```python
from build123d import *

# Parameters (mm, degrees)
SKETCH1_R           = 1.75
BOSS_EXTRUDE1_DEPTH = 5
FILLET1_R           = 5
CUT_EXTRUDE1_DEPTH  = 10
SKETCH3_R           = 1.75
CUT_EXTRUDE2_DEPTH  = 10


with BuildPart() as part:
    # Sketch1 → Boss-Extrude1 (new body)
    with BuildSketch(Plane(origin=(0, 0, 0), x_dir=(1, 0, 0), z_dir=(0, 1, 0))):
        with BuildLine():
            Line((-15, 0), (-15, 50))
            ThreePointArc((-15, 50), (0, 65), (15, 50))
            Line((15, 50), (15, 0))
            ThreePointArc((15, 0), (0, -15), (-15, 0))
        make_face()
        Circle(SKETCH1_R, mode=Mode.SUBTRACT)
        with BuildLine():
            Line((12.25773045, 35.509501863), (8.623388818, 27.715631082))
            Line((8.623388818, 27.715631082), (10.414213562, 25.924806337))
            ThreePointArc((10.414213562, 25.924806337), (10.414213562, 23.096379213), (7.585786438, 23.096379213))
            Line((7.585786438, 23.096379213), (4.804718696, 25.877446954))
            ThreePointArc((4.804718696, 25.877446954), (4.249316753, 26.944364161), (4.406316685, 28.13689704))
            Line((4.406316685, 28.13689704), (8.632499302, 37.19997491))
            ThreePointArc((8.632499302, 37.19997491), (11.2903514, 38.167353961), (12.25773045, 35.509501863))
        make_face(mode=Mode.SUBTRACT)
    extrude(amount=BOSS_EXTRUDE1_DEPTH)

    # Fillet1
    fillet1_edges = [part.edges().sort_by_distance(p)[0] for p in [
        (8.623388818, 2.5, -27.715631082),
    ]]
    fillet(fillet1_edges, radius=FILLET1_R)

    # Sketch2 → Cut-Extrude1 (cut)
    with BuildSketch(Plane(origin=(0, 5, 0), x_dir=(1, 0, 0), z_dir=(0, 1, 0))):
        with BuildLine():
            Line((-15, 26.324644949), (-40.925594741, 69.238213195))
            Line((-40.925594741, 69.238213195), (-58.771967888, 111.080687023))
            Line((-58.771967888, 111.080687023), (39.28439299, 102.825794629))
            Line((39.28439299, 102.825794629), (15, 36.046990739))
            ThreePointArc((15, 36.046990739), (14.81014445, 39.245839168), (14.243243524, 42.399773179))
            ThreePointArc((14.243243524, 42.399773179), (11.621838426, 46.208407589), (7.127072402, 47.292169164))
            ThreePointArc((7.127072402, 47.292169164), (-0.175202385, 45.163669538), (-6.484026655, 40.9148504))
            ThreePointArc((-6.484026655, 40.9148504), (-11.826766868, 34.252893813), (-15, 26.324644949))
        make_face()
    extrude(amount=-CUT_EXTRUDE1_DEPTH, mode=Mode.SUBTRACT)

    # Sketch3 → Cut-Extrude2 (cut)
    with BuildSketch(Plane(origin=(0, 5, 0), x_dir=(1, 0, 0), z_dir=(0, 1, 0))):
        with Locations((-1.301778952, 33.126107378)):
            Circle(SKETCH3_R)
        with Locations((-2.207127715, 39.057409395)):
            Circle(SKETCH3_R)
        with Locations((-7.905919506, 31.519764857)):
            Circle(SKETCH3_R)
    extrude(amount=-CUT_EXTRUDE2_DEPTH, mode=Mode.SUBTRACT)


solid = part.part
```
The listing builds one solid part. Answer for the finished solid, in the listing's coordinates (mm). A direction names the side the tool comes from. Coordinates: 2 decimals unless noted, no trailing zeros. Write each loop counter-clockwise with the first axis right and the second up, starting at its lowest first coordinate (ties: lowest second). Pieces come first, ordered by that corner, then holes.
Q1. The mould has two halves that part along X. Classify faces 1 (the cylindrical face through (-1.53, 2.54, -34.86)), 2 (the flat face through (0, 0, -17)), 3 (the flat face through (-15, 2, -13)): released by +X, released by -X, zero draft, split by the parting line, or undercut.
Returned:
face 1: undercut
face 2: zero draft
face 3: released by -X
Q2. Section B-B, the plane y = 3.15 is taken. Give the number of separate pieces and of enclosed holes in the cut face, then the cut area to 3 significant figures.
Returned:
separate pieces: 1
enclosed holes: 5
area: 1,520 mm2
Q3. Section C-C, the plane x = -11 is taken. Write down the section's boundary in (y, z), then the cut area to 3 significant figures.
Returned:
outline: (0, -35.59) - (5, -35.59) - (5, 10.2) - (0, 10.2) - close
area: 229 mm2
Q4. Section A-A, the plane x = -7.5 is taken. Write down the section's boundary in (y, z), then the cut area to 3 significant figures.
Returned:
outline: (0, -39.93) - (5, -39.93) - (5, -33.22) - (0, -33.22) - close; (0, -29.82) - (5, -29.82) - (5, 12.99) - (0, 12.99) - close
area: 248 mm2
Q5. Find the intervals of material crossed by line 1 along X through (y, z) = (1, 1); line 2 along Z through (x, y) = (1, 1.3); line 3 along X through (y, z) = (1.25, -32), in increasing order.
Returned:
line 1: x = -14.97 to -1.44, 1.44 to 14.97
line 2: z = -45.68 to -1.44, 1.44 to 14.97
line 3: x = -13.01 to -9.59, -6.22 to -2.64, 0.04 to 6.21, 10.62 to 15
Q6. Which of the six approach directions +Z, -Z, +X, -X, +Y, -Y give full straight-line access (tool end or side, diameter ignored) to faces 4 (the flat face through (6.21, 2.46, -24.47)), 5 (the flat face through (0, 5, -17))?
Returned:
face 4: +Y, -Y
face 5: +Z, -Z, +X, -X, +Y
